Verification items for the finished model (mm, model axes). A direction names the side the tool comes from. Give positions to 0.01 mm unless a question says otherwise; leave off trailing zeros. Write each loop counter-clockwise with the first axis right and the second up, starting at its lowest first coordinate (ties: lowest second). Pieces come first, ordered by that corner, then holes. Notation, with made-up numbers: (-16, 76) - (21, 76) arc R12 ccw to (21, 90) - close; hole circle Ø10 at (-16.5, 58). An arc over 180 degrees is marked (long way). Put each result on its own line as item: value.
from build123d import *

# Parameters (mm, degrees)
SKETCH1_R           = 4.5
SKETCH1_R_2         = 4.2
BOSS_EXTRUDE1_DEPTH = 1.7
SKETCH2_R           = 4.5
SKETCH2_R_2         = 3.3
BOSS_EXTRUDE2_DEPTH = 0.3
CHAMFER1_SIZE       = 0.15
CHAMFER2_SIZE       = 0.15


with BuildPart() as part:
    # Sketch1 → Boss-Extrude1 (new body)
    with BuildSketch(Plane(origin=(0, 0, 0), x_dir=(1, 0, 0), z_dir=(0, 1, 0))):
        with Locations(Location((0, 0, 0), (0, 0, 270))):
            Circle(SKETCH1_R)
        with Locations(Location((0, 0, 0), (0, 0, 270))):
            Circle(SKETCH1_R_2, mode=Mode.SUBTRACT)
    extrude(amount=BOSS_EXTRUDE1_DEPTH)

    # Sketch2 → Boss-Extrude2 (add)
    with BuildSketch(Plane(origin=(0, 1.7, 0), x_dir=(1, 0, 0), z_dir=(0, 1, 0))):
        with Locations(Location((0, 0, 0), (0, 0, 270))):
            Circle(SKETCH2_R)
        with Locations(Location((0, 0, 0), (0, 0, 270))):
            Circle(SKETCH2_R_2, mode=Mode.SUBTRACT)
    extrude(amount=BOSS_EXTRUDE2_DEPTH)

    # Chamfer1
    chamfer1_edges = [part.edges().sort_by_distance(p)[0] for p in [
        (0, 2, -4.5),
    ]]
    chamfer(chamfer1_edges, length=CHAMFER1_SIZE)

    # Chamfer2
    chamfer2_edges = [part.edges().sort_by_distance(p)[0] for p in [
        (0, 1.7, -4.2),
    ]]
    chamfer(chamfer2_edges, length=CHAMFER2_SIZE)

    # Mirror1: part across plane


with BuildPart() as part_1:
    add(part.part)
    add(part.part.mirror(Plane.ZX))


solid = part_1.part
Q1. Set-up check for faces 3 (the face through (-3, -1.7, -2)), 4 (the face through (3, -2, 2)): record each of +Z, -Z, +X, -X, +Y, -Y from which the full face is reachable in a straight line by a thin tool's end or side.
Answers follow:
face 3: none
face 4: +Z, -Z, +X, -X, -Y
Q2. Go/stop test with flat-tipped pins: pin 1 Ø4 at (x, z) = (1, -0.5) entering from -Y; pin 2 Ø1.5 at (y, z) = (-0.5, -3.5) entering from +X; pin 3 Ø4 at (x, z) = (-1.5, -1) entering from +Y. Record where each tip stops, or that it passes through.
Answers follow:
pin 1: passes through
pin 2: stops at x = 3.56
pin 3: stops at y = 2
Q3. Section check C-C, the plane y = -1.05. Record the cut outline in (x, z), plus the area to 3 significant figures.
Answers follow:
outline: circle Ø9 at (0, 0); hole circle Ø8.4 at (0, 0)
area: 8.20 mm2
Q4. Release check for a two-part mould opening along X. For faces 1 (the face through (3, 2, 2)), 2 (the face through (-3.22, -1.85, -0.72)) record: released by +X, released by -X, zero draft, split by the parting line, or undercut.
Answers follow:
face 1: zero draft
face 2: undercut
Q5. Section check A-A, the plane x = 0. Record the cut outline in (y, z), plus the area to 3 significant figures.
Answers follow:
outline: (-2, -4.35) - (-1.85, -4.5) - (1.85, -4.5) - (2, -4.35) - (2, -3.3) - (1.7, -3.3) - (1.7, -4.05) - (1.55, -4.2) - (-1.55, -4.2) - (-1.7, -4.05) - (-1.7, -3.3) - (-2, -3.3) - close; (-2, 3.3) - (-1.7, 3.3) - (-1.7, 4.05) - (-1.55, 4.2) - (1.55, 4.2) - (1.7, 4.05) - (1.7, 3.3) - (2, 3.3) - (2, 4.35) - (1.85, 4.5) - (-1.85, 4.5) - (-2, 4.35) - close
area: 3.48 mm2
Q6. Scan lines: line 1 along X through (y, z) = (1.8, 0); line 2 along Y through (x, z) = (-1, -3.75); line 3 along X through (y, z) = (1.1, 0). Record each from-to range of solid material in increasing order.
Answers follow:
line 1: x = -4.5 to -3.3, 3.3 to 4.5
line 2: y = -2 to -1.7, 1.7 to 2
line 3: x = -4.5 to -4.2, 4.2 to 4.5
Q7. Section check B-B, the plane z = 0. Record the cut outline in (x, y), plus the area to 3 significant figures.
Answers follow:
outline: (-4.5, -1.85) - (-4.35, -2) - (-3.3, -2) - (-3.3, -1.7) - (-4.05, -1.7) - (-4.2, -1.55) - (-4.2, 1.55) - (-4.05, 1.7) - (-3.3, 1.7) - (-3.3, 2) - (-4.35, 2) - (-4.5, 1.85) - close; (3.3, -2) - (4.35, -2) - (4.5, -1.85) - (4.5, 1.85) - (4.35, 2) - (3.3, 2) - (3.3, 1.7) - (4.05, 1.7) - (4.2, 1.55) - (4.2, -1.55) - (4.05, -1.7) - (3.3, -1.7) - close
area: 3.48 mm2
